Model file for the job. Use its own axes, mm. A direction names the side the tool comes from. Coordinates: 2 decimals unless noted, no trailing zeros. Order: outer loops, then holes, each group sorted by start corner. A loop starts at its lowest first (then second) coordinate and runs counter-clockwise, first axis right, second up. Notation, with made-up numbers: (-23.5, 86.5) - (0.5, 86.5) arc R30 cw to (0.5, 112.5) - close; hole circle Ø10 at (71, 57). An arc over 180 degrees is marked (long way). Put each result on its own line as item: value. Start each with the question number.
```python
from build123d import *

# Parameters (mm, degrees)
SKETCH1_R           = 2
BOSS_EXTRUDE1_DEPTH = 6
FILLET1_R           = 2


with BuildPart() as part:
    # Sketch1 → Boss-Extrude1 (new body)
    with BuildSketch(Plane.XY):
        with BuildLine():
            Line((28.912721374, 2.543366015), (3.087278626, 2.543366015))
            ThreePointArc((3.087278626, 2.543366015), (1.706829801, 3.617558849), (0, 4))
            ThreePointArc((0, 4), (-4, 0), (0, -4))
            ThreePointArc((0, -4), (1.706829801, -3.617558849), (3.087278626, -2.543366015))
            Line((3.087278626, -2.543366015), (28.912721374, -2.543366015))
            ThreePointArc((28.912721374, -2.543366015), (30.293170199, -3.617558849), (32, -4))
            ThreePointArc((32, -4), (36, 0), (32, 4))
            ThreePointArc((32, 4), (30.293170199, 3.617558849), (28.912721374, 2.543366015))
        make_face()
        Circle(SKETCH1_R, mode=Mode.SUBTRACT)
        with Locations((32, 0)):
            Circle(SKETCH1_R, mode=Mode.SUBTRACT)
    extrude(amount=BOSS_EXTRUDE1_DEPTH)

    # Fillet1
    fillet1_edges = [part.edges().sort_by_distance(p)[0] for p in [
        (28.912721374, 2.543366015, 3),
        (28.912721374, -2.543366015, 3),
        (3.087278626, -2.543366015, 3),
        (3.087278626, 2.543366015, 3),
    ]]
    fillet(fillet1_edges, radius=FILLET1_R)


solid = part.part
```
Item 1: Flat gauge pins, fed straight in: pin 1 Ø2.5 at (x, y) = (32, 0) entering from +Z; pin 2 Ø3 at (x, z) = (19.5, 3.5) entering from -Y; pin 3 Ø1.5 at (y, z) = (1.5, 4.5) entering from +X; pin 4 Ø2 at (x, z) = (7.5, 2.5) entering from +Y. Where does each tip first touch, or does it go through?
Item 2: Pull direction Y, two halves, no side cores. Call faces 4 (the face through (3.213, -2.672, 3.042)), 5 (the face through (16, 0, 6)), 6 (the face through (3.231, 2.665, 3.042)), 7 (the face through (0, -2, 3)): pulls with the +Y half, pulls with the -Y half, needs draft (parallel to the pull), parting line crosses it, or undercut.
Item 3: Slice it at C-C, the plane x = 28.5. Give the cut face in (y, z).
Item 4: Slice it at A-A, the plane z = 3.45. Give the cut face in (x, y), plus the area to 3 significant figures.
Item 5: 3-axis set-ups, long thin cutter, end or side, ignore diameter. For faces 1 (the face through (33.847, -0.766, 2.958)), 2 (the face through (16, 2.543, 3)), 3 (the face through (16, -2.543, 3)): which of +Z, -Z, +X, -X, +Y, -Y reach the whole face in a straight line?
Item 6: Wall check: line 1 along X through (y, z) = (-1.5, 3.6); line 2 along X through (y, z) = (-1, 2.05); line 3 along Y through (x, z) = (32, 3.3). Give the ranges that are in metal, low to high.
Item 7: Slice it at D-D, the plane y = 1.25. Give the cut face in (x, z).
Item 8: Slice it at B-B, the plane y = -1.5. Give the cut face in (x, z), plus the area to 3 significant figures.
Here are the results:
1. pin 1: passes through
1. pin 2: stops at y = -2.54
1. pin 3: stops at x = 35.93
1. pin 4: stops at y = 2.54
2. face 4: pulls with the -Y half
2. face 5: needs draft
2. face 6: pulls with the +Y half
2. face 7: undercut
3. outline: (-2.59, 0) - (2.59, 0) - (2.59, 6) - (-2.59, 6) - close
4. outline: (2.61, -3.03) arc R2 cw to (3.92, -2.54) - (28.08, -2.54) arc R2 cw to (29.39, -3.03) arc R4 ccw (long way) to (29.39, 3.03) arc R2 cw to (28.08, 2.54) - (3.92, 2.54) arc R2 cw to (2.61, 3.03) arc R4 ccw (long way) to start; hole circle Ø4 at (0, 0); hole circle Ø4 at (32, 0)
4. area: 201 mm^2
5. face 1: +Z, -Z
5. face 2: +Z, -Z, +Y
5. face 3: +Z, -Z, -Y
6. line 1: x = -3.71 to -1.32, 1.32 to 30.68, 33.32 to 35.71
6. line 2: x = -3.87 to -1.73, 1.73 to 30.27, 33.73 to 35.87
6. line 3: y = -4 to -2, 2 to 4
7. outline: (-3.8, 0) - (-1.56, 0) - (-1.56, 6) - (-3.8, 6) - close; (1.56, 0) - (30.44, 0) - (30.44, 6) - (1.56, 6) - close; (33.56, 0) - (35.8, 0) - (35.8, 6) - (33.56, 6) - close
8. outline: (-3.71, 0) - (-1.32, 0) - (-1.32, 6) - (-3.71, 6) - close; (1.32, 0) - (30.68, 0) - (30.68, 6) - (1.32, 6) - close; (33.32, 0) - (35.71, 0) - (35.71, 6) - (33.32, 6) - close
8. area: 205 mm^2
